Geometry: see drawing. Coordinates: mm, zero at the bounding-box minimum. A direction names the side the tool comes from. Give positions to 0.01 mm unless a question says otherwise; leave off trailing zeros. Loops run counter-clockwise (first coordinate to the right, second up) from the corner with the lowest first, then second, coordinate; pieces in that order, holes last. Notation, with made-up numbers: (31.5, -24) -> (62.5, -24) arc R13 ccw to (62.5, -20) -> close; hole circle Ø2 at (44.5, 63.5). An arc over 180 degrees is marked (long way). Return JSON: item names as keys, results as strings. Group by question number.
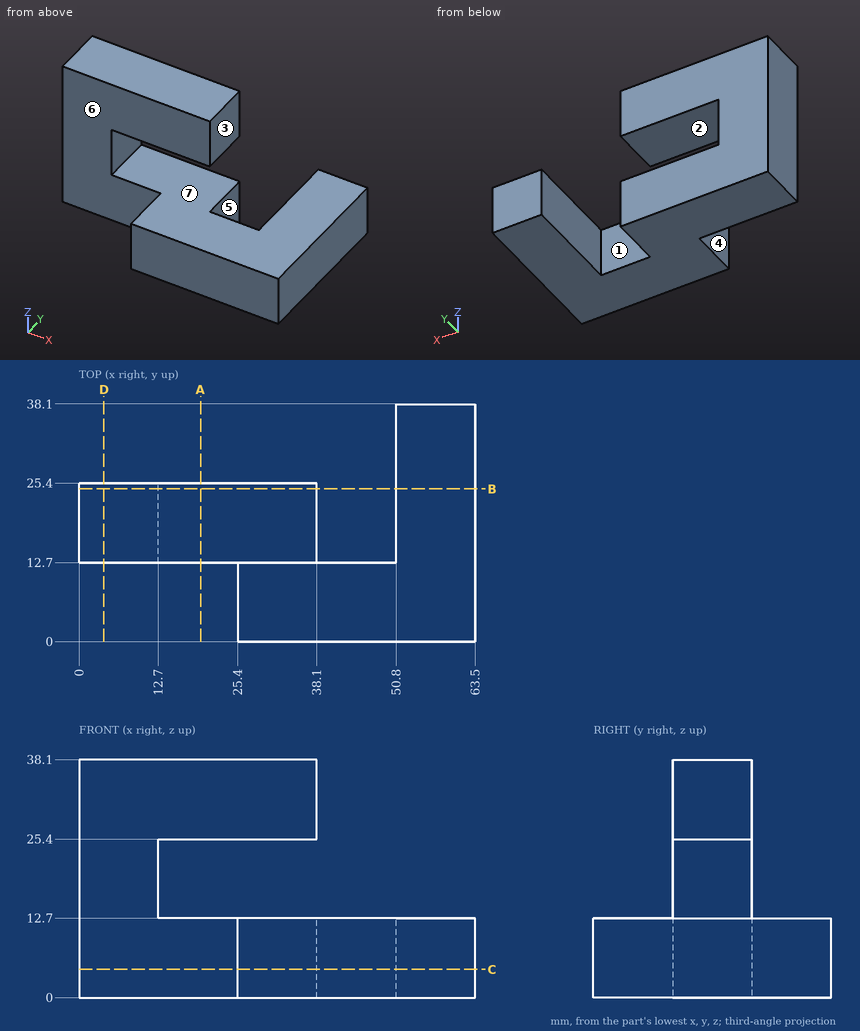
1) Cut plane C-C on z = 4.5. Return loops of the section in (x, y), then the cut area to 3 significant figures.
2) Material intervals for line 1 (X direction, y = 17, z = 10.5); line 2 (Z direction, x = 52.5, y = 21); line 3 (X direction, y = 35.5, z = 7.5), sorted ascending.
3) Reachability of the marked faces 4, 5, 6 and 7 from +Z, -Z, +X, -X, +Y, -Y: full face, straight path, thin tool, end or side. Return the list, or none.
4) Cut plane A-A on x = 19.5. Return loops of the section in (y, z).
5) Cut plane D-D on x = 4. Return loops of the section in (y, z), then the cut area to 3 significant figures.
6) Contact query for flat-ended pins moving along their axis: P1, Ø4, axis at y = 31.5, z = 5.5, coming from the -X side; P2, Ø10, axis at y = 19.5, z = 34.5, coming from the +X side; P3, Ø6.5, axis at y = 21.5, z = 16, coming from the +X side. Output: stop coordinate, or through.
7) Mould query, pull axis X, two halves, no side actions, for the marked faces 1, 2 and 3. Classes: released by +X, released by -X, zero draft, split by the parting line, or undercut.
8) Cut plane B-B on y = 24.5. Return loops of the section in (x, z).
Calculated:
{
 "1": {"outline": "(0, 12.7) -> (25.4, 12.7) -> (25.4, 0) -> (63.5, 0) -> (63.5, 38.1) -> (50.8, 38.1) -> (50.8, 12.7) -> (38.1, 12.7) -> (38.1, 25.4) -> (0, 25.4) -> close", "area": "1,290 mm2"},
 "2": {"line 1": "0 to 38.1, 50.8 to 63.5", "line 2": "0 to 12.7", "line 3": "50.8 to 63.5"},
 "3": {"face 4": "+Z, -Z, -X, -Y", "face 5": "+Z, -Z, +Y", "face 6": "+Z, -X, -Y", "face 7": "+X, +Y, -Y"},
 "4": {"outline": "(12.7, 0) -> (25.4, 0) -> (25.4, 12.7) -> (12.7, 12.7) -> close; (12.7, 25.4) -> (25.4, 25.4) -> (25.4, 38.1) -> (12.7, 38.1) -> close"},
 "5": {"outline": "(12.7, 0) -> (25.4, 0) -> (25.4, 38.1) -> (12.7, 38.1) -> close", "area": "484 mm2"},
 "6": {"P1": "x = 50.8", "P2": "x = 38.1", "P3": "x = 12.7"},
 "7": {"face 1": "undercut", "face 2": "zero draft", "face 3": "released by +X"},
 "8": {"outline": "(0, 0) -> (38.1, 0) -> (38.1, 12.7) -> (12.7, 12.7) -> (12.7, 25.4) -> (38.1, 25.4) -> (38.1, 38.1) -> (0, 38.1) -> close; (50.8, 0) -> (63.5, 0) -> (63.5, 12.7) -> (50.8, 12.7) -> close"}
}
